from build123d import *

# Parameters (mm, degrees)
SKETCH2_W                      = 30
SKETCH2_H                      = 15
BOSS_EXTRUDE1_DEPTH            = 6
CBORE_FOR_M4_SHCS1_D           = 4.8
CBORE_FOR_M4_SHCS1_CBORE_D     = 8
CBORE_FOR_M4_SHCS1_CBORE_DEPTH = 4
BOSS_EXTRUDE2_DEPTH            = 30
CUT_EXTRUDE1_START             = -15
SKETCH6_W                      = 5.3
SKETCH6_H                      = 20.435085946
SKETCH6_H_2                    = 17.047451378
CUT_EXTRUDE1_DEPTH             = 28.107006543
FILLET1_R                      = 4
CBORE_FOR_M3_SHCS1_D           = 3.6
CBORE_FOR_M3_SHCS1_CBORE_D     = 6.5
CBORE_FOR_M3_SHCS1_CBORE_DEPTH = 3


with BuildPart() as part:
    # Sketch2 → Boss-Extrude1 (new body)
    with BuildSketch(Plane.XY):
        with Locations((15, 7.5)):
            Rectangle(SKETCH2_W, SKETCH2_H)
    extrude(amount=BOSS_EXTRUDE1_DEPTH)

    # CBORE for M4 SHCS1 (through all)
    with Locations(Plane.XY.offset(6)):
        with Locations((7.5, 7.5), (22.5, 7.5)):
            CounterBoreHole(CBORE_FOR_M4_SHCS1_D / 2, CBORE_FOR_M4_SHCS1_CBORE_D / 2, CBORE_FOR_M4_SHCS1_CBORE_DEPTH)

    # Sketch5 → Boss-Extrude2 (add)
    with BuildSketch(Plane(origin=(30, 0, 0), x_dir=(0, 0, -1), z_dir=(1, 0, 0))):
        with BuildLine():
            Line((0, 0), (-2, -7))
            ThreePointArc((-2, -7), (-9.236067977, -11.472135955), (-10, -3))
            Line((-10, -3), (-6, 0))
            Line((-6, 0), (0, 0))
        make_face()
    extrude(amount=-BOSS_EXTRUDE2_DEPTH)

    # Sketch6 → Cut-Extrude1 (cut, through all)
    with BuildSketch(Plane(origin=(0, 15, 0), x_dir=(1, 0, 0), z_dir=(0, 1, 0)).offset(CUT_EXTRUDE1_START)):
        with Locations((20.65, -5.918041099)):
            Rectangle(SKETCH6_W, SKETCH6_H)
        with Locations((9.65, -5.207730625)):
            Rectangle(SKETCH6_W, SKETCH6_H_2)
    extrude(amount=-CUT_EXTRUDE1_DEPTH, mode=Mode.SUBTRACT)

    # Fillet1
    # the kernel refuses this fillet: 4 mm, written as the material it takes off along each edge
    with BuildSketch(Plane(origin=(26, 11, 2), x_dir=(0, 0, 1), z_dir=(0, 1, 0))) as fillet1_piece_1_section:
        Polygon((0, 0), (FILLET1_R, 0), (FILLET1_R, FILLET1_R), (0, FILLET1_R), align=None)
    fillet1_piece_1 = extrude(amount=FILLET1_R, mode=Mode.PRIVATE)
    fillet1_piece_1 = fillet1_piece_1 - Plane(origin=(26, 11, 2), x_dir=(-0.7071067811865475, 0, -0.7071067811865475), z_dir=(0, 1, 0)) * Sphere(FILLET1_R, mode=Mode.PRIVATE)
    add(fillet1_piece_1, mode=Mode.SUBTRACT)
    with BuildSketch(Plane(origin=(4, 11, 2), x_dir=(0, 1, 0), z_dir=(-1, 0, 0))) as fillet1_piece_2_section:
        Polygon((0, 0), (FILLET1_R, 0), (FILLET1_R, -FILLET1_R), (0, -FILLET1_R), align=None)
    fillet1_piece_2 = extrude(amount=FILLET1_R, mode=Mode.PRIVATE)
    fillet1_piece_2 = fillet1_piece_2 - Plane(origin=(4, 11, 2), x_dir=(0, -0.7071067811865475, -0.7071067811865475), z_dir=(-1, 0, 0)) * Sphere(FILLET1_R, mode=Mode.PRIVATE)
    add(fillet1_piece_2, mode=Mode.SUBTRACT)
    with BuildSketch(Plane(origin=(30, -10, 6), x_dir=(-1, 0, 0), z_dir=(0, 1, 0))) as fillet1_piece_3_section:
        with BuildLine():
            CenterArc((FILLET1_R, -FILLET1_R), FILLET1_R, 90, 90)
            Line((0, -FILLET1_R), (0, 0))
            Line((0, 0), (FILLET1_R, 0))
        make_face()
    fillet1_piece_3 = extrude(amount=21, mode=Mode.PRIVATE)
    fillet1_piece_3 = split(fillet1_piece_3, bisect_by=Plane(origin=(29.062495656, 2.503698405, 2.66173546), z_dir=(0, 0.8, 0.6)), keep=Keep.TOP, mode=Mode.PRIVATE)
    add(fillet1_piece_3, mode=Mode.SUBTRACT)
    with BuildSketch(Plane(origin=(26, 15, 6), x_dir=(0, 0, -1), z_dir=(-1, 0, 0))) as fillet1_piece_4:
        with BuildLine():
            CenterArc((FILLET1_R, FILLET1_R), FILLET1_R, 180, 90)
            Line((0, FILLET1_R), (0, 0))
            Line((0, 0), (FILLET1_R, 0))
        make_face()
    extrude(amount=22, mode=Mode.SUBTRACT)
    with BuildSketch(Plane(origin=(0, 11, 6), x_dir=(0, 0, -1), z_dir=(0, -1, 0))) as fillet1_piece_5_section:
        with BuildLine():
            CenterArc((FILLET1_R, FILLET1_R), FILLET1_R, 180, 90)
            Line((0, FILLET1_R), (0, 0))
            Line((0, 0), (FILLET1_R, 0))
        make_face()
    fillet1_piece_5 = extrude(amount=21, mode=Mode.PRIVATE)
    fillet1_piece_5 = split(fillet1_piece_5, bisect_by=Plane(origin=(0.937504344, 2.503698405, 2.66173546), z_dir=(0, 0.8, 0.6)), keep=Keep.TOP, mode=Mode.PRIVATE)
    add(fillet1_piece_5, mode=Mode.SUBTRACT)
    with BuildSketch(Plane(origin=(0, 15, -10), x_dir=(0, -1, 0), z_dir=(0, 0, 1)), Plane(origin=(30, 15, -10), x_dir=(-1, 0, 0), z_dir=(0, 0, 1))) as fillet1_piece_6:
        with BuildLine():
            CenterArc((FILLET1_R, FILLET1_R), FILLET1_R, 180, 90)
            Line((0, FILLET1_R), (0, 0))
            Line((0, 0), (FILLET1_R, 0))
        make_face()
    extrude(amount=12, mode=Mode.SUBTRACT)

    # CBORE for M3 SHCS1 (through all)
    with Locations(Plane.ZY):
        with Locations((7, -7)):
            CounterBoreHole(CBORE_FOR_M3_SHCS1_D / 2, CBORE_FOR_M3_SHCS1_CBORE_D / 2, CBORE_FOR_M3_SHCS1_CBORE_DEPTH)


solid = part.part
CAD build for the part. Positions are in the model's coordinates, mm. A direction names the side the tool comes from. Round coordinates to 2 decimals unless told otherwise and drop trailing zeros. Loops run counter-clockwise (first coordinate to the right, second up) from the corner with the lowest first, then second, coordinate; pieces in that order, holes last. Notation, with made-up numbers: (76.5, 30.5) - (120.5, 30.5) arc R21 ccw to (120.5, 40.5) - close; hole circle Ø5 at (-18, 11.5). An arc over 180 degrees is marked (long way). Put each result on its own line as item: value.
1. Pin check, flat tips, straight feed: P1, Ø8, axis at x = 3.5, y = 4.5, coming from the +Z side; P2, Ø2, axis at y = -8.5, z = 6.5, coming from the -X side; P3, Ø2, axis at x = 21, z = 3.5, coming from the -Y side; P4, Ø3, axis at x = 22.5, y = 7.5, coming from the -Z side. Stop position of each tip, or through.
Geometry check:
P1: z = 6
P2: x = 3
P3: y = 0
P4: through
2. Two-plate mould, pull along Y, no slides. Class faces 1 (the flat face through (18, -5, 6)), 2 (the flat face through (10, 0, 3)), 3 (the cylindrical face through (1.479, -4.803, 4.605)): released by +Y, released by -Y, zero draft, split by the parting line, or undercut.
Geometry check:
face 1: zero draft
face 2: released by -Y
face 3: undercut
3. Slice it at A-A on y = -6. List the corners of the cut face in (x, z).
Geometry check:
outline: (0, 1.71) - (7, 1.71) - (7, 5.5) - (3, 5.5) - (3, 3.91) - (0, 3.91) - close; (0, 10.09) - (3, 10.09) - (3, 8.5) - (7, 8.5) - (7, 11.9) - (0, 11.9) - close; (12.3, 1.71) - (18, 1.71) - (18, 5.5) - (12.3, 5.5) - close; (12.3, 8.5) - (18, 8.5) - (18, 11.9) - (12.3, 11.9) - close; (23.3, 1.71) - (30, 1.71) - (30, 5.5) - (23.3, 5.5) - close; (23.3, 8.5) - (30, 8.5) - (30, 11.9) - (23.3, 11.9) - close
4. Slice it at C-C on y = 8.25. List the corners of the cut face in (x, z).
Geometry check:
outline: (0, 0) - (5.22, 0) - (5.22, 2) - (3.57, 2) - (3.57, 5.98) arc R4 ccw to (0, 2) - close; (9.78, 0) - (20.22, 0) - (20.22, 2) - (18.57, 2) - (18.57, 6) - (11.43, 6) - (11.43, 2) - (9.78, 2) - close; (24.78, 0) - (30, 0) - (30, 2) arc R4 ccw to (26.43, 5.98) - (26.43, 2) - (24.78, 2) - close
5. 3-axis set-ups, long thin cutter, end or side, ignore diameter. For faces 4 (the cylindrical face through (28.797, 5.423, 4.859)), 5 (the cylindrical face through (19.3, 5.1, 4)), 6 (the flat face through (21, 0, 3)), 7 (the flat face through (3.5, -3.5, 1)), 8 (the flat face through (15, 4, 6)): which of +Z, -Z, +X, -X, +Y, -Y reach the whole face in a straight line?
Geometry check:
face 4: +Z, +X, +Y
face 5: +Z
face 6: +Z, -Z, -Y
face 7: -Z, +X, -X, -Y
face 8: +Z, +X, -X, +Y
6. Slice it at B-B on x = 16.5. List the corners of the cut face in (y, z).
Geometry check:
outline: (-7, 2) - (0, 0) - (15, 0) - (15, 2) arc R4 ccw to (11, 6) - (0, 6) - (-3, 10) arc R5 ccw (long way) to start; hole circle Ø3.6 at (-7, 7)
7. Slice it at D-D on z = 8.25. List the corners of the cut face in (x, y).
Geometry check:
outline: (0, -11.84) - (7, -11.84) - (7, -8.3) - (3, -8.3) - (3, -10) - (0, -10) - close; (0, -4) - (3, -4) - (3, -5.7) - (7, -5.7) - (7, -1.69) - (0, -1.69) - close; (12.3, -11.84) - (18, -11.84) - (18, -8.3) - (12.3, -8.3) - close; (12.3, -5.7) - (18, -5.7) - (18, -1.69) - (12.3, -1.69) - close; (23.3, -11.84) - (30, -11.84) - (30, -8.3) - (23.3, -8.3) - close; (23.3, -5.7) - (30, -5.7) - (30, -1.69) - (23.3, -1.69) - close
8. Wall check: line 1 (X direction, y = -5.75, z = 4.75); line 2 (X direction, y = -9.5, z = 4.75); line 3 (Z direction, x = 24, y = -7.75). Give the ranges that are in metal, low to high.
Geometry check:
line 1: 3 to 7, 12.3 to 18, 23.3 to 30
line 2: 0 to 7, 12.3 to 18, 23.3 to 30
line 3: 2.06 to 5.36, 8.64 to 11.94
